Check sheet for the modelled part. Datum: model origin and axes. Units: mm. A direction names the side the tool comes from. Give positions to 0.01 mm unless a question says otherwise; leave off trailing zeros. Order: outer loops, then holes, each group sorted by start corner. A loop starts at its lowest first (then second) coordinate and runs counter-clockwise, first axis right, second up. Notation, with made-up numbers: (41.25, 40) -> (50.25, 40) arc R20 ccw to (50.25, 72) -> close; hole circle Ø7 at (-19.75, -1.5). An arc over 180 degrees is marked (long way). One line per question, with ' | ' between items. Start each with the question number.
Autodesk Inventor part; units mm, degrees
ref_plane "YZ Plane" through (0, 0, 0) normal (1, 0, 0) x (0, 1, 0)
ref_plane "XZ Plane" through (0, 0, 0) normal (0, 1, 0) x (-1, 0, 0)
ref_plane "XY Plane" through (0, 0, 0) normal (0, 0, 1) x (1, 0, 0)
sketch "Sketch1" plane through (0, 0, 0) normal (0, 1, 0) x (-1, 0, 0)
  line L0 (0, 0) -> (0, 15)
  line L1 (0, 15) -> (14.1421, 15)
  line L2 (14.1421, 15) -> (14.1421, 0)
  line L3 (14.1421, 0) -> (0, -14.1421)
  line L4 (0, -14.1421) -> (-15, -14.1421)
  line L5 (-15, -14.1421) -> (-15, 0)
  line L6 (-15, 0) -> (0, 0)
  dimension "d0" = 15
  dimension "d1" = 10
extrude "Extrusion1" add sketch "Sketch1" along normal blind 151
chamfer "Chamfer1" distance 10 angle 45 2 edges at (-14.1421, 75.5, 15) (15, 75.5, -14.1421)
sketch "Sketch2" plane through (0, 151, 0) normal (0, 1, 0) x (1, 0, 0)
  line L0 (5, 14.1421) -> (15, 4.1421)
  line L1 (5, 14.1421) -> (0, 14.1421)
  line L2 (0, 14.1421) -> (-14.1421, 0)
  line L3 (-14.1421, 0) -> (-14.1421, -5)
  line L4 (-4.1421, -15) -> (-14.1421, -5)
  line L5 (-4.1421, -15) -> (0, -15)
  line L6 (0, -15) -> (0, 0)
  line L7 (0, 0) -> (15, 0)
  line L8 (15, 0) -> (15, 4.1421)
  circle A0 centre (-39.9264, 39.9264) radius 11.15
  line L9 (5, 14.1421) -> (-37.4264, 56.5685)
  line L10 (-37.4264, 56.5685) -> (-42.4264, 56.5685)
  line L11 (-42.4264, 56.5685) -> (-56.5685, 42.4264)
  line L12 (-56.5685, 42.4264) -> (-56.5685, 37.4264)
  line L13 (-56.5685, 37.4264) -> (-14.1421, -5)
  line L14 (-4.1421, -15) -> (-14.1421, -5)
  line L15 (5, 14.1421) -> (15, 4.1421)
  line L16 (-14.1421, 0) -> (-14.1421, -5)
  dimension "d7" = 22.3
  dimension "d8" = 60
  dimension "d9" = 27.0711
  dimension "d10" = 13.5355
  dimension "d11" = 13.5355
extrude "Extrusion2" add sketch "Sketch2" against normal blind 10 contours L1 L2 L3 L13 L12 L11 L10 L9
sketch "Sketch3" plane through (0, 151, 0) normal (0, 1, 0) x (1, 0, 0)
  circle A0 centre (-39.9264, 39.9264) radius 11.15
  circle A1 centre (-39.9264, 39.9264) radius 9.15
  point P0 (0, 0)
  dimension "d14" = 2
extrude "Extrusion3" add sketch "Sketch3" against normal blind 2
sketch "Sketch4" plane through (-14.1421, 0, 0) normal (-1, 0, 0) x (0, 0, 1)
  line L0 (5, 141) -> (0, 141)
  line L1 (0, 0) -> (0, 141)
  line L2 (0, 0) -> (5, 0)
  line L3 (5, 141) -> (5, 0)
  line L4 (-37.4264, 151) -> (15, 151)
  line L5 (-37.4264, 151) -> (-37.4264, 141)
  line L6 (5, 141) -> (-37.4264, 141)
  line L7 (5, 141) -> (5, 0)
  line L8 (5, 0) -> (15, 0)
  line L9 (15, 0) -> (15, 151)
  point P0 (0, 0)
  point P1 (7.5, 40)
  point P2 (7.5, 111)
  dimension "d17" = 7.5
  dimension "d18" = 40
  dimension "d19" = 40
hole "Hole1" at (-14.1421, 40, 7.5) at (-14.1421, 111, 7.5) direction (1, 0, 0) diameter 3.6 end through all counterbore diameter 6.5 counterbore depth 10
sketch "Sketch5" plane through (5, 0, -14.1421) normal (0, 0, -1) x (-1, 0, 0)
  line L0 (5, 141) -> (0, 141)
  line L1 (0, 0) -> (0, 141)
  line L2 (0, 0) -> (5, 0)
  line L3 (5, 0) -> (5, 141)
  line L4 (-10, 151) -> (42.4264, 151)
  line L5 (-10, 151) -> (-10, 0)
  line L6 (-10, 0) -> (0, 0)
  line L7 (0, 0) -> (0, 141)
  line L8 (42.4264, 141) -> (0, 141)
  line L9 (42.4264, 151) -> (42.4264, 141)
  point P0 (-2.5, 40)
  point P1 (-2.5, 111)
  dimension "d27" = 7.5
  dimension "d28" = 40
  dimension "d29" = 40
hole "Hole2" at (7.5, 40, -14.1421) at (7.5, 111, -14.1421) direction (0, 0, 1) diameter 3.6 end through all counterbore diameter 6.5 counterbore depth 10
sketch "Sketch6" plane through (0, 0, -14.1421) normal (-0.7071, 0, -0.7071) x (-0.7071, 0, 0.7071)
  circle A0 centre (10, -125) radius 3
  circle A1 centre (10, -85) radius 3
  circle A2 centre (10, -45) radius 3
  circle A3 centre (10, -5) radius 3
  circle A4 centre (10, 35) radius 3
  circle A5 centre (10, 75) radius 3
  circle A6 centre (10, 115) radius 3
  circle A7 centre (10, 135) radius 3
  circle A8 centre (10, 95) radius 3
  circle A9 centre (10, 55) radius 3
  circle A10 centre (10, 15) radius 3
  circle A11 centre (10, -25) radius 3
  circle A12 centre (10, -65) radius 3
  circle A13 centre (10, -105) radius 3
  circle A14 centre (10, -145) radius 3
  line L0 (14.5, 140) -> (5.5, 140)
  line L1 (5.5, 140) -> (5.5, -210)
  line L2 (14.5, -210) -> (5.5, -210)
  line L3 (14.5, 140) -> (14.5, -210)
  circle A15 centre (10, -205) radius 3
  circle A16 centre (10, -165) radius 3
  circle A17 centre (10, -185) radius 3
  point P0 (10, 0)
hole "Hole3" at (-7.0711, 15, -7.0711) at (-7.0711, 35, -7.0711) at (-7.0711, 55, -7.0711) at (-7.0711, 75, -7.0711) at (-7.0711, 95, -7.0711) at (-7.0711, 115, -7.0711) at (-7.0711, 135, -7.0711) direction (0.7071, 0, 0.7071) diameter 2.8 end through all
equation "\"d10\" = 0.5 * d9"
equation "\"d11\" = d10"
properties part number "Corner Z Brace w Bearing" material "ABS Plastic"
1. Cross-section at A-A on z = -44.5. Record the boundary of the cut face in (x, y).
2. Cross-section at C-C on y = 111. Record the boundary of the cut face in (x, z).
3. Cross-section at B-B on z = 7.5. Record the boundary of the cut face in (x, y).
4. Tool access check on faces 1 (the face through (-4.142, 41.4, 8.9)), 2 (the face through (4.278, 110.577, -7.961)), 3 (the face through (-7.17, 69.51, -6.97)), 4 (the face through (-14.142, 70, 3)). Record the directions out of +Z, -Z, +X, -X, +Y, -Y that give a thin tool (end or side, any length) a straight path to the whole face; none if there is none.
5. Mould release check, pull along Y, two halves, no side actions. Record for faces 5 (the face through (-21, 151, -21)), 6 (the face through (2, 70, -14.142)), 7 (the face through (8.9, 112.4, -4.142)), 8 (the face through (-3, 0, -3)): +Y half, -Y half, draft (parallel to the pull), parting line (faces both ways), or undercut.
6. Cross-section at D-D on x = 7.5. Record the boundary of the cut face in (y, z).
7. Scan lines: probe 1 along Y at (x, z) = (7.5, -2.15); probe 2 along Y at (x, z) = (7, -3); probe 3 along X at (y, z) = (111, -7.25). Record each from-to range of solid material in increasing order.
8. Go/stop test with flat-tipped pins: pin 1 (12 mm diameter, centred on x = -12.5, y = 131, fed in from -Z); pin 2 (1.5 mm diameter, centred on x = 1.5, y = 100, fed in from -Z); pin 3 (2 mm diameter, centred on y = 25.5, z = -13.5, fed in from -X). Record where each tip stops, or that it passes through.
Response values:
1) outline: (-54.49, 141) -> (-50.1, 141) -> (-50.1, 149) -> (-47.85, 149) -> (-47.85, 151) -> (-54.49, 151) -> close; (-32, 149) -> (-29.76, 149) -> (-29.76, 141) -> (-25.36, 141) -> (-25.36, 151) -> (-32, 151) -> close
2) outline: (-14.14, 0) -> (0, -14.14) -> (4.25, -14.14) -> (4.25, -4.14) -> (5.7, -4.14) -> (5.7, 0) -> (0, 0) -> (0, 5.7) -> (-4.14, 5.7) -> (-4.14, 4.25) -> (-14.14, 4.25) -> close; (-8.39, 10.75) -> (-4.14, 10.75) -> (-4.14, 9.3) -> (0, 9.3) -> (0, 15) -> (-4.14, 15) -> close; (9.3, -4.14) -> (10.75, -4.14) -> (10.75, -8.39) -> (15, -4.14) -> (15, 0) -> (9.3, 0) -> close
3) outline: (-11.64, 0) -> (0, 0) -> (0, 38.2) -> (-4.14, 38.2) -> (-4.14, 36.75) -> (-11.64, 36.75) -> close; (-11.64, 43.25) -> (-4.14, 43.25) -> (-4.14, 41.8) -> (0, 41.8) -> (0, 109.2) -> (-4.14, 109.2) -> (-4.14, 107.75) -> (-11.64, 107.75) -> close; (-11.64, 114.25) -> (-4.14, 114.25) -> (-4.14, 112.8) -> (0, 112.8) -> (0, 151) -> (-11.64, 151) -> close
4) face 1: -X | face 2: -Z | face 3: -Z, -X, -Y | face 4: +Z, -Z, -X, -Y
5) face 5: +Y half | face 6: draft | face 7: undercut | face 8: -Y half
6) outline: (0, -11.64) -> (36.75, -11.64) -> (36.75, -4.14) -> (38.2, -4.14) -> (38.2, 0) -> (0, 0) -> close; (41.8, -4.14) -> (43.25, -4.14) -> (43.25, -11.64) -> (107.75, -11.64) -> (107.75, -4.14) -> (109.2, -4.14) -> (109.2, 0) -> (41.8, 0) -> close; (112.8, -4.14) -> (114.25, -4.14) -> (114.25, -11.64) -> (151, -11.64) -> (151, 0) -> (112.8, 0) -> close
7) probe 1: y = 0 to 38.2, 41.8 to 109.2, 112.8 to 151 | probe 2: y = 0 to 38.27, 41.73 to 109.27, 112.73 to 151 | probe 3: x = -6.89 to 4.25, 10.75 to 11.89
8) pin 1: stops at z = -7.64 | pin 2: stops at z = -14.14 | pin 3: stops at x = -1.64
